The listing builds one solid part. Answer for the finished solid, in the listing's coordinates (mm). Face numbers are marked on the shaded views. A direction names the side the tool comes from. Coordinates: 2 decimals unless noted, no trailing zeros. Order: outer loops, then holes, each group sorted by start corner. A loop starts at its lowest first (then second) coordinate and runs counter-clockwise, first axis right, second up. Notation, with made-up numbers: (41, 15) -> (82, 15) arc R25 cw to (82, 32) -> close; hole circle Ø2 at (19, 9). An arc over 180 degrees is marked (long way). One line per question, with ' | ' between items.
from build123d import *

# Parameters (mm, degrees)
BOSS_EXTRUDE1_DEPTH = 3
SKETCH1_R           = 6
BOSS_EXTRUDE3_DEPTH = 2
SKETCH4_R           = 1.5
CUT_EXTRUDE1_DEPTH  = 46.914811248
SKETCH5_R           = 4
CUT_EXTRUDE2_DEPTH  = 2
CUT_EXTRUDE3_DEPTH  = 46.914811248


with BuildPart() as part:
    # Sketch3 → Boss-Extrude1 (new body)
    with BuildSketch(Plane(origin=(0, 0, 0), x_dir=(1, 0, 0), z_dir=(0, 1, 0))):
        Polygon((-10, 16.53279569), (-10, -6.048583789), (34.799193535, -29.53279569), (34.799193535, -6.951416211), align=None)
    extrude(amount=BOSS_EXTRUDE1_DEPTH)

    # Sketch1 → Boss-Extrude3 (add)
    with BuildSketch(Plane(origin=(0, 0, 0), x_dir=(1, 0, 0), z_dir=(0, 1, 0))):
        with Locations(Location((0, 0, 0), (0, 0, 270))):
            Circle(SKETCH1_R)
        with Locations(Location((24.799193535, -13, 0), (0, 0, 270))):
            Circle(SKETCH1_R)
    extrude(amount=-BOSS_EXTRUDE3_DEPTH)

    # Sketch4 → Cut-Extrude1 (cut, through all)
    with BuildSketch(Plane(origin=(0, 3, 0), x_dir=(1, 0, 0), z_dir=(0, 1, 0))):
        with Locations(Location((0, 0, 0), (0, 0, 270))):
            Circle(SKETCH4_R)
        with Locations(Location((24.799193535, -13, 0), (0, 0, 270))):
            Circle(SKETCH4_R)
    extrude(amount=-CUT_EXTRUDE1_DEPTH, mode=Mode.SUBTRACT)

    # Sketch5 → Cut-Extrude2 (cut)
    with BuildSketch(Plane(origin=(0, 3, 0), x_dir=(1, 0, 0), z_dir=(0, 1, 0))):
        with Locations(Location((0, 0, 0), (0, 0, 270))):
            Circle(SKETCH5_R)
        with Locations(Location((24.799193535, -13, 0), (0, 0, 270))):
            Circle(SKETCH5_R)
    extrude(amount=-CUT_EXTRUDE2_DEPTH, mode=Mode.SUBTRACT)

    # Sketch7 → Cut-Extrude3 (cut, through all)
    with BuildSketch(Plane(origin=(0, 3, 0), x_dir=(1, 0, 0), z_dir=(0, 1, 0))):
        Polygon((-10, 16.53279569), (-10, 12.53279569), (-2.369478912, 12.53279569), align=None)
        Polygon((34.799193535, -29.53279569), (34.799193535, -25.53279569), (27.168672447, -25.53279569), align=None)
    extrude(amount=-CUT_EXTRUDE3_DEPTH, mode=Mode.SUBTRACT)


solid = part.part
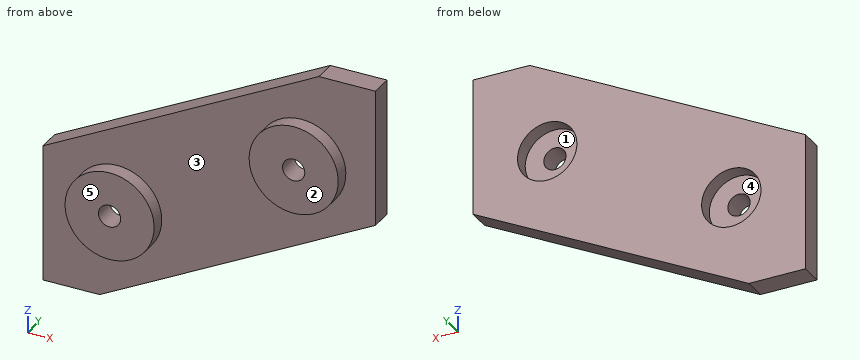
Item 1: Section B-B, the plane x = 0 is taken. Give the vertices of the cut face in (y, z).
Computed values:
outline: (-2, -6) -> (0, -6) -> (0, -11.29) -> (3, -11.29) -> (3, -4) -> (1, -4) -> (1, -1.5) -> (-2, -1.5) -> close; (-2, 1.5) -> (1, 1.5) -> (1, 4) -> (3, 4) -> (3, 11.29) -> (0, 11.29) -> (0, 6) -> (-2, 6) -> close
Item 2: Determine the mould class of the marked faces 4 and 5 for opening direction X: pulls with the +X half, pulls with the -X half, needs draft (parallel to the pull), parting line crosses it, or undercut.
Computed values:
face 4: undercut | face 5: needs draft
Item 3: Section A-A, the plane z = 13 is taken. Give the vertices of the cut face in (x, y), plus the area to 3 significant figures.
Computed values:
outline: (3.26, 0) -> (18.8, 0) -> (18.8, -2) -> (23.3, -2) -> (23.3, 1) -> (20.8, 1) -> (20.8, 3) -> (3.26, 3) -> close; (26.3, -2) -> (30.8, -2) -> (30.8, 0) -> (34.8, 0) -> (34.8, 3) -> (28.8, 3) -> (28.8, 1) -> (26.3, 1) -> close | area: 93.6 mm^2
Item 4: For the marked faces 1, 2 and 3, determine the directions among +Z, -Z, +X, -X, +Y, -Y from which every point of the face is accessible in a straight line to the end or side of a thin tool.
Computed values:
face 1: +Y | face 2: +Z, -Z, +X, -X, -Y | face 3: -Y
Item 5: Each of these flat-tipped pins is pushed along its axis until it touches: pin 1 Ø5 at (x, z) = (24.8, 13) entering from +Y; pin 2 Ø9 at (x, z) = (-1, -2) entering from +Y; pin 3 Ø6 at (x, z) = (13, 11) entering from -Y. Where does it stop, or does it pass through?
Computed values:
pin 1: stops at y = 1 | pin 2: stops at y = 3 | pin 3: stops at y = 0
Item 6: Section C-C, the plane x = 22 is taken. Give the vertices of the cut face in (y, z), plus the area to 3 significant figures.
Computed values:
outline: (-2, 7.69) -> (0, 7.69) -> (0, 0.24) -> (3, 0.24) -> (3, 10.14) -> (1, 10.14) -> (1, 15.86) -> (3, 15.86) -> (3, 22.82) -> (0, 22.82) -> (0, 18.31) -> (-2, 18.31) -> close | area: 77.5 mm^2
Item 7: Section D-D, the plane y = -0.5 is taken. Give the vertices of the cut face in (x, z), plus the area to 3 significant figures.
Computed values:
outline: circle Ø12 at (0, 0); circle Ø12 at (24.8, 13); hole circle Ø3 at (0, 0); hole circle Ø3 at (24.8, 13) | area: 212 mm^2
Item 8: Find the intervals of material crossed by L1, parallel to Y at x = 24, z = 15.5; L2, parallel to Y at x = 11, z = 11; L3, parallel to Z at x = -0.5, y = 1.65, in increasing order.
Computed values:
L1: y = -2 to 1 | L2: y = 0 to 3 | L3: z = -11.55 to -3.97, 3.97 to 11.03
